from build123d import *

# Parameters (mm, degrees)
SKETCH_1_R               = 10
EXTRUDE_2_DEPTH          = 32
CUT_EXTRUDE_1_DEPTH      = 35.985711369
CUT_EXTRUDE_1_DEPTH_BACK = 35.985711369
SKETCH_3_W               = 8
SKETCH_3_H               = 26
CUT_EXTRUDE_2_DEPTH      = 35.985711369
CUT_EXTRUDE_2_DEPTH_BACK = 35.985711369
SKETCH_4_W               = 2
SKETCH_4_H               = 32
SKETCH_5_R               = 1.25
CUT_EXTRUDE_3_DEPTH      = 35.467375879
CUT_EXTRUDE_4_DEPTH      = 35.467375879
CUT_EXTRUDE_4_DEPTH_BACK = 35.467375879
SKETCH_6_R               = 2


with BuildPart() as part:
    # 草图1 → 凸台-拉伸2 (new body)
    with BuildSketch(Plane.XY):
        Circle(SKETCH_1_R)
    extrude(amount=EXTRUDE_2_DEPTH)

    # 草图3 → 切除-拉伸1 (cut, two sides: drawn at the far end of the back side and taken through both)
    with BuildSketch(Plane(origin=(0, 0, 0), x_dir=(1, 0, 0), z_dir=(0, 1, 0)).offset(-CUT_EXTRUDE_1_DEPTH_BACK)):
        with Locations((0, -19)):
            Rectangle(SKETCH_3_W, SKETCH_3_H)
    extrude(amount=CUT_EXTRUDE_1_DEPTH + CUT_EXTRUDE_1_DEPTH_BACK, mode=Mode.SUBTRACT)

    # 草图4 → 切除-拉伸2 (cut, two sides: drawn at the far end of the back side and taken through both)
    with BuildSketch(Plane(origin=(0, 0, 0), x_dir=(1, 0, 0), z_dir=(0, 1, 0)).offset(-CUT_EXTRUDE_2_DEPTH_BACK)):
        with Locations((-9, -16)):
            Rectangle(SKETCH_4_W, SKETCH_4_H)
        with Locations((9, -16)):
            Rectangle(SKETCH_4_W, SKETCH_4_H)
    extrude(amount=CUT_EXTRUDE_2_DEPTH + CUT_EXTRUDE_2_DEPTH_BACK, mode=Mode.SUBTRACT)

    # 草图5 → 切除-拉伸3 (cut, through all)
    with BuildSketch(Plane(origin=(0, 0, 0), x_dir=(-1, 0, 0), z_dir=(0, 0, -1))):
        with Locations((0, 7)):
            Circle(SKETCH_5_R)
        with Locations((0, -7)):
            Circle(SKETCH_5_R)
    extrude(amount=-CUT_EXTRUDE_3_DEPTH, mode=Mode.SUBTRACT)

    # 草图6 → 切除-拉伸4 (cut, two sides: drawn at the far end of the back side and taken through both)
    with BuildSketch(Plane(origin=(0, 0, 0), x_dir=(0, 0, -1), z_dir=(1, 0, 0)).offset(-CUT_EXTRUDE_4_DEPTH_BACK)):
        with Locations((-23, 0)):
            Circle(SKETCH_6_R)
    extrude(amount=CUT_EXTRUDE_4_DEPTH + CUT_EXTRUDE_4_DEPTH_BACK, mode=Mode.SUBTRACT)


solid = part.part
Can you work these out from the model? Positions are in its coordinate system, mm. A direction names the side the tool comes from. Round coordinates to 2 decimals unless told otherwise and drop trailing zeros. Loops run counter-clockwise (first coordinate to the right, second up) from the corner with the lowest first, then second, coordinate; pieces in that order, holes last. Notation, with made-up numbers: (9, -31.5) - (60, -31.5) arc R27 ccw to (60, -12.5) - close; hole circle Ø7 at (-19.75, 25.25). An arc over 180 degrees is marked (long way). Answer in a Markdown table with one row per item. Add a question column.
Q1. For pin 1 Ø3 at (x, y) = (-2, 0) entering from +Z, with a flat end and sliding along its axis, tell me the tip position at first contact or that it passes through.
Q2. I want a section at B-B on x = 0. List the corners of the cut face in (y, z) for me.
Q3. I want a section at A-A on z = 23. List the corners of the cut face in (x, y) for me, and give its area (3 significant figures).
Q4. I want a section at D-D on y = 7. List the corners of the cut face in (x, z) for me.
Q5. Which directions (+Z, -Z, +X, -X, +Y, -Y) give clear straight access to the entire face, cutting with the end or side of a thin tool? Please do faces 4 (the flat face through (4, 0, 19)), 5 (the cylindrical face through (6, -1.2, 24.6)).
Q6. I need wall thicknesses on L1, parallel to Y at x = 0, z = 2.5; L2, parallel to X at y = -0.5, z = 15; L3, parallel to Y at x = 6, z = 23. Which ranges of each line are inside material? Lowest first, please.
Q7. We'd pull the mould along Y, two halves only. Please class faces 1 (the flat face through (-6, 0, 32)), 2 (the cylindrical face through (6, 8, 12)), 3 (the cylindrical face through (0.27, -8.22, 2.96)): pulls with the +Y half, pulls with the -Y half, needs draft (parallel to the pull), parting line crosses it, or undercut.
Q8. I want a section at C-C on z = 13.5. List the corners of the cut face in (x, y) for me, and give its area (3 significant figures).
A:
| question | item | result |
|---|---|---|
| 1 | pin 1 | z = 6 |
| 2 | outline | (-10, 0) - (-8.25, 0) - (-8.25, 6) - (-10, 6) - close; (-5.75, 0) - (5.75, 0) - (5.75, 6) - (-5.75, 6) - close; (8.25, 0) - (10, 0) - (10, 6) - (8.25, 6) - close |
| 3 | outline | (-8, -6) arc R10 ccw to (-4, -9.17) - (-4, -2) - (-8, -2) - close; (-8, 2) - (-4, 2) - (-4, 9.17) arc R10 ccw to (-8, 6) - close; (4, -9.17) arc R10 ccw to (8, -6) - (8, -2) - (4, -2) - close; (4, 2) - (8, 2) - (8, 6) arc R10 ccw to (4, 9.17) - close |
| 3 | area | 93.8 mm^2 |
| 4 | outline | (-7.14, 0) - (-1.25, 0) - (-1.25, 6) - (-4, 6) - (-4, 32) - (-7.14, 32) - close; (1.25, 0) - (7.14, 0) - (7.14, 32) - (4, 32) - (4, 6) - (1.25, 6) - close |
| 5 | face 4 | +Z, +Y, -Y |
| 5 | face 5 | +X, -X |
| 6 | L1 | -10 to -8.25, -5.75 to 5.75, 8.25 to 10 |
| 6 | L2 | -8 to -4, 4 to 8 |
| 6 | L3 | -8 to -2, 2 to 8 |
| 7 | face 1 | needs draft |
| 7 | face 2 | pulls with the +Y half |
| 7 | face 3 | undercut |
| 8 | outline | (-8, -6) arc R10 ccw to (-4, -9.17) - (-4, 9.17) arc R10 ccw to (-8, 6) - close; (4, -9.17) arc R10 ccw to (8, -6) - (8, 6) arc R10 ccw to (4, 9.17) - close |
| 8 | area | 126 mm^2 |
